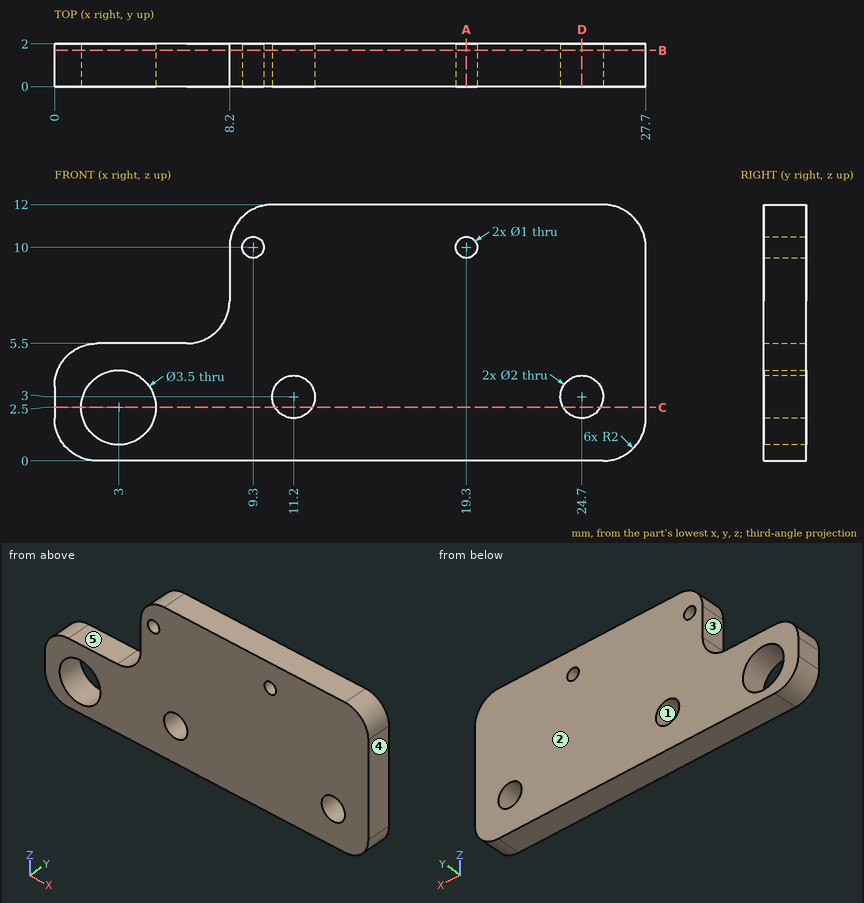
Design review of the part shown in the three views and the two pictorial views. Dimensions are in mm from the part's minimum x, y and z. A direction names the side the tool comes from. Round coordinates to 2 decimals unless told otherwise and drop trailing zeros. Write each loop counter-clockwise with the first axis right and the second up, starting at its lowest first coordinate (ties: lowest second). Pieces come first, ordered by that corner, then holes.
Item 1: We need section C-C on z = 2.5. Write out the cut boundary in (x, y).
Item 2: We need section B-B on y = 1.7. Write out the cut boundary in (x, z).
Item 3: For the marked faces 4 and 5, list the 3-axis set-ups (+Z, -Z, +X, -X, +Y, -Y) from which the entire face can be reached by the end or side of a thin tool; tool diameter is ignored.
Item 4: We need section D-D on x = 24.7. Write out the cut boundary in (y, z), and give its area (3 significant figures).
Item 5: Clearance check with flat-ended pins moving along their axes: pin 1 Ø0.6 at (y, z) = (1, 9) entering from -X; pin 2 Ø1.8 at (x, z) = (24.7, 3) entering from -Y. State where each tip first meets the part, or that it passes through.
Item 6: The part is to be moulded in two halves that separate along X. For the marked faces 1, 2 and 3, say which applies: +X half, -X half, draft (parallel to the pull), parting line (faces both ways), or undercut.
Item 7: We need section A-A on x = 19.3. Write out the cut boundary in (y, z).
Item 8: For probe 1 along X at (y, z) = (1.4, 2.5); probe 2 along Z at (x, y) = (24, 1.1); probe 3 along X at (y, z) = (1.8, 8.5), list the stretches that pass through material, from the lowest coordinate up.
Returned:
1. outline: (0, 0) - (1.25, 0) - (1.25, 2) - (0, 2) - close; (4.75, 0) - (10.33, 0) - (10.33, 2) - (4.75, 2) - close; (12.07, 0) - (23.83, 0) - (23.83, 2) - (12.07, 2) - close; (25.57, 0) - (27.7, 0) - (27.7, 2) - (25.57, 2) - close
2. outline: (0, 2) arc R2 ccw to (2, 0) - (25.7, 0) arc R2 ccw to (27.7, 2) - (27.7, 10) arc R2 ccw to (25.7, 12) - (10.2, 12) arc R2 ccw to (8.2, 10) - (8.2, 7.5) arc R2 cw to (6.2, 5.5) - (2, 5.5) arc R2 ccw to (0, 3.5) - close; hole circle Ø3.5 at (3, 2.5); hole circle Ø1 at (9.3, 10); hole circle Ø2 at (11.2, 3); hole circle Ø1 at (19.3, 10); hole circle Ø2 at (24.7, 3)
3. face 4: +Z, -Z, +X, +Y, -Y
3. face 5: +Z, -X, +Y, -Y
4. outline: (0, 0) - (2, 0) - (2, 2) - (0, 2) - close; (0, 4) - (2, 4) - (2, 12) - (0, 12) - close
4. area: 20.0 mm2
5. pin 1: stops at x = 8.2
5. pin 2: passes through
6. face 1: undercut
6. face 2: draft
6. face 3: -X half
7. outline: (0, 0) - (2, 0) - (2, 9.5) - (0, 9.5) - close; (0, 10.5) - (2, 10.5) - (2, 12) - (0, 12) - close
8. probe 1: x = 0 to 1.25, 4.75 to 10.33, 12.07 to 23.83, 25.57 to 27.7
8. probe 2: z = 0 to 2.29, 3.71 to 12
8. probe 3: x = 8.2 to 27.7
